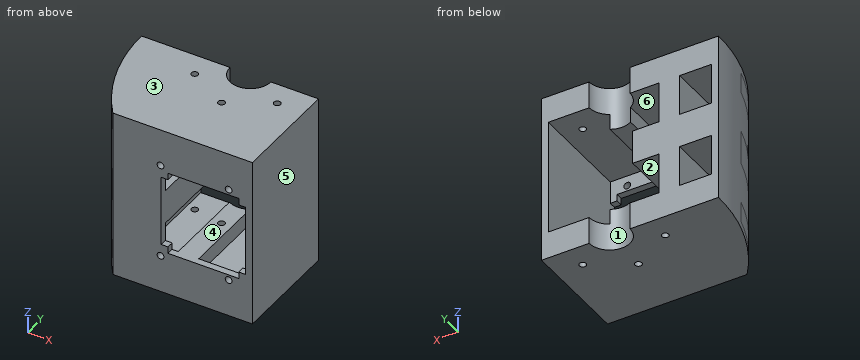
Autodesk Inventor part; units mm, degrees
ref_plane "YZ Plane" through (0, 0, 0) normal (1, 0, 0) x (0, 1, 0)
ref_plane "XZ Plane" through (0, 0, 0) normal (0, 1, 0) x (-1, 0, 0)
ref_plane "XY Plane" through (0, 0, 0) normal (0, 0, 1) x (1, 0, 0)
sketch "Sketch1" plane through (0, 0, 0) normal (0, 0, 1) x (1, 0, 0)
  circle A0 centre (0, 80) radius 130 construction
  line L0 (0, -50) -> (0, 0) construction
  line L1 (0, 0) -> (-102.4695, 0) construction
  arc A1 (-130, 80) -> (-102.4695, 0) centre (0, 80) ccw
  line L2 (-130, 80) -> (0, 80)
  line L3 (0, 80) -> (0, 0)
  line L4 (-102.4695, 0) -> (0, 0)
  dimension "d0" = 260
  dimension "d1" = 50
extrude "Extrusion1" add sketch "Sketch1" along normal blind 125
sketch "Sketch6" plane through (-130, 80, 0) normal (0, 1, 0) x (1, 0, 0)
  line L0 (0, 0) -> (0, -125)
  line L1 (0, 0) -> (130, 0)
  line L2 (130, 0) -> (130, -125)
  line L3 (130, -125) -> (0, -125)
  line L4 (0, -125) -> (0, 0)
  line L5 (5, -120) -> (125, -120)
  line L6 (125, -120) -> (125, -5)
  line L7 (125, -5) -> (5, -5)
  line L8 (5, -5) -> (5, -120)
  point P0 (130, 0)
  dimension "d25" = 5
extrude "Extrusion5" cut sketch "Sketch6" against normal blind 75 contours L8 L7 L6 L5
sketch "Sketch7" plane through (-102.4695, 0, 0) normal (0, -1, 0) x (1, 0, 0)
  circle A0 centre (35, 97.53) radius 2.5
  circle A1 centre (85, 97.53) radius 2.5
  line L0 (0, 125) -> (102.4695, 125)
  line L1 (0, 0) -> (0, 125)
  circle A2 centre (35, 27.53) radius 2.5
  circle A3 centre (85, 27.53) radius 2.5
  line L2 (102.4695, 0) -> (102.4695, 125)
  dimension "d28" = 5
  dimension "d29" = 5
  dimension "d30" = 27.47
  dimension "d31" = 50
  dimension "d33" = 5
  dimension "d34" = 5
  dimension "d35" = 70
  dimension "d82" = 35
extrude "Extrusion6" cut sketch "Sketch7" against normal through all
sketch "Sketch8" plane through (0, 0, 125) normal (0, 0, 1) x (1, 0, 0)
  line L0 (0, 80) -> (-130, 80)
  arc A0 (-130, 80) -> (-102.4695, 0) centre (0, 80) ccw
  arc A1 (-130, 80) -> (-102.4695, 0) centre (9.9581, 83.4269) ccw
  line L1 (-102.4695, 0) -> (-97.4695, 0)
  line L2 (-102.4695, 0) -> (0, 0)
  line L3 (-130, 80) -> (-125, 80)
  arc A2 (-125, 80) -> (-97.4695, 0) centre (14.9581, 83.4269) ccw
  dimension "d40" = 5
  dimension "d41" = 5
  dimension "d42" = 140
extrude "Extrusion7" add sketch "Sketch8" against normal blind 125
sketch "Sketch11" plane through (-130, 5, 0) normal (0, 1, 0) x (1, 0, 0)
  line L0 (125, -5) -> (125, -120)
  line L1 (125, -50) -> (5, -50)
  line L2 (5, -50) -> (5, -65)
  line L3 (5, -65) -> (125, -65)
  line L4 (125, -65) -> (125, -50)
  line L5 (125, -60) -> (5, -60)
  line L6 (5, -60) -> (5, -75)
  line L7 (5, -75) -> (125, -75)
  line L8 (125, -75) -> (125, -60)
  line L9 (32.7619, 0) -> (32.7619, -150)
  line L10 (125, -105) -> (5, -105)
  line L11 (5, -105) -> (5, -120)
  line L12 (5, -120) -> (125, -120)
  line L13 (125, -120) -> (125, -105)
  line L14 (125, -20) -> (5, -20)
  line L15 (5, -20) -> (5, -5)
  line L16 (5, -5) -> (125, -5)
  line L17 (125, -5) -> (125, -20)
  line L18 (5, -5) -> (125, -5)
  line L19 (5, -120) -> (5, -5)
  line L20 (125, -120) -> (5, -120)
  line L21 (125, -5) -> (125, -20)
  point P0 (130, 0)
  point P1 (65, -120)
  point P2 (65, -5)
  point P3 (5, -12.5)
  point P4 (5, -57.5)
  dimension "d54" = 15
  dimension "d55" = 15
  dimension "d56" = 15
  dimension "d57" = 15
  dimension "d58" = 30
  dimension "d59" = 30
  dimension "d66" = 5
extrude "Extrusion10" add sketch "Sketch11" along normal blind 75 contours L0 L14 L9 L16 | L9 L14 L15 L16 | L0 L5 L9 L1 | L0 L3 L9 L5 | L9 L5 L2 L1 | L0 L7 L9 L3 | L9 L3 L2 L5 | L9 L7 L6 L3 | L0 L12 L9 L10 | L9 L12 L11 L10
sketch "Sketch12" plane through (-130, 5, 0) normal (0, 1, 0) x (1, 0, 0)
  line L0 (27.5305, 0) -> (130, 0)
  line L1 (27.5305, -125) -> (130, -125)
  line L2 (72.5, 0) -> (87.5, 0)
  line L3 (87.5, 0) -> (87.5, -125)
  line L4 (87.5, -125) -> (72.5, -125)
  line L5 (72.5, -125) -> (72.5, 0)
  line L6 (28.5256, 0) -> (43.5256, 0)
  line L7 (43.5256, 0) -> (43.5256, -125)
  line L8 (43.5256, -125) -> (28.5256, -125)
  line L9 (28.5256, -125) -> (28.5256, 0)
  line L10 (130, 0) -> (130, -125)
  dimension "d62" = 15
  dimension "d63" = 15
  dimension "d92" = 42.5
extrude "Extrusion11" add sketch "Sketch12" along normal blind 75 contours L0 L7 L1 L9 | L0 L3 L1 L5
sketch "Sketch9" plane through (0, 0, 125) normal (0, 0, 1) x (1, 0, 0)
  circle A0 centre (-50, 80) radius 15
  point P0 (0, 0)
  point P1 (0, 80)
  dimension "d45" = 30
  dimension "d46" = 50
extrude "Extrusion8" cut sketch "Sketch9" against normal through all
sketch "Sketch13" plane through (0, 0, 0) normal (0, 0, -1) x (-1, 0, 0)
  arc A0 (102.4695, 0) -> (130, 80) centre (-9.9581, 83.4269) ccw
  line L0 (130, 80) -> (130, 80)
  arc A1 (102.4695, 0) -> (130, 80) centre (0, 80) ccw
  line L1 (130, 80) -> (130, 80)
  line L2 (65, 80) -> (130, 80)
  line L3 (130, 80) -> (130, 0)
  line L4 (130, 0) -> (102.4695, 0)
  point P0 (0, 0)
  dimension "d67" = 140
extrude "Extrusion12" cut sketch "Sketch13" against normal through all contours A1 L3 L4
sketch "Sketch14" plane through (0, 0, 125) normal (0, 0, 1) x (1, 0, 0)
  line L0 (-102.4695, 0) -> (0, 0) construction
  line L1 (-50, 0) -> (-50, 196.0469) construction
  line L2 (0, 80) -> (-93.0222, 80) construction
  line L3 (-50, 80) -> (28.9192, 80) construction
  circle A0 centre (-50, 115) radius 2.5
  circle A1 centre (-50, 80) radius 35 construction
  circle A2 centre (-80.3109, 97.5) radius 2.5
  circle A3 centre (-80.3109, 62.5) radius 2.5
  circle A4 centre (-50, 45) radius 2.5
  circle A5 centre (-19.6891, 62.5) radius 2.5
  circle A6 centre (-19.6891, 97.5) radius 2.5
  dimension "d74" = 70
  dimension "d70" = 50
  dimension "d72" = 5
  dimension "d77" = 360
extrude "Extrusion13" cut sketch "Sketch14" against normal through all contours A3 | A4 | A5
sketch "Sketch16" plane through (-102.4695, 0, 0) normal (0, -1, 0) x (1, 0, 0)
  line L0 (35.4695, 31.5) -> (35.4695, 93.5) construction
  line L1 (97.4695, 93.5) -> (35.4695, 93.5) construction
  line L2 (35.4695, 93.5) -> (35.4695, 31.5) construction
  line L3 (35.4695, 31.5) -> (97.4695, 31.5) construction
  line L4 (97.4695, 31.5) -> (97.4695, 93.5) construction
  line L5 (0, 125) -> (102.4695, 125)
  line L6 (0, 0) -> (102.4695, 0)
  line L7 (102.4695, 0) -> (102.4695, 125)
  line L8 (97.4695, 93.5) -> (92.4695, 93.5) construction
  line L9 (92.4695, 93.5) -> (92.4695, 88.5) construction
  line L10 (92.4695, 88.5) -> (97.4695, 88.5) construction
  line L11 (97.4695, 88.5) -> (97.4695, 93.5) construction
  line L12 (35.4695, 31.5) -> (40.4695, 31.5) construction
  line L13 (40.4695, 31.5) -> (40.4695, 36.5) construction
  line L14 (40.4695, 36.5) -> (35.4695, 36.5) construction
  line L15 (35.4695, 36.5) -> (35.4695, 31.5) construction
  line L16 (35.4695, 93.5) -> (40.4695, 93.5) construction
  line L17 (40.4695, 93.5) -> (40.4695, 88.5) construction
  line L18 (40.4695, 88.5) -> (35.4695, 88.5) construction
  line L19 (35.4695, 88.5) -> (35.4695, 93.5) construction
  line L20 (97.4695, 31.5) -> (92.4695, 31.5) construction
  line L21 (92.4695, 31.5) -> (92.4695, 36.5) construction
  line L22 (92.4695, 36.5) -> (97.4695, 36.5) construction
  line L23 (97.4695, 36.5) -> (97.4695, 31.5) construction
  line L24 (92.4695, 93.5) -> (40.4695, 93.5)
  line L25 (40.4695, 88.5) -> (40.4695, 93.5)
  line L26 (35.4695, 88.5) -> (40.4695, 88.5)
  line L27 (35.4695, 88.5) -> (35.4695, 36.5)
  line L28 (35.4695, 36.5) -> (40.4695, 36.5)
  line L29 (40.4695, 36.5) -> (40.4695, 31.5)
  line L30 (40.4695, 31.5) -> (92.4695, 31.5)
  line L31 (92.4695, 31.5) -> (92.4695, 36.5)
  line L32 (92.4695, 36.5) -> (97.4695, 36.5)
  line L33 (97.4695, 20) -> (97.4695, 50)
  line L34 (97.4695, 36.5) -> (97.4695, 88.5)
  line L35 (97.4695, 75) -> (97.4695, 105)
  line L36 (92.4695, 88.5) -> (97.4695, 88.5)
  line L37 (92.4695, 88.5) -> (92.4695, 93.5)
  point P0 (97.4695, 62.5)
  point P1 (102.4695, 62.5)
  point P2 (66.4695, 31.5)
  point P3 (51.2348, 0)
  dimension "d100" = 62
  dimension "d101" = 62
  dimension "d102" = 5
  dimension "d103" = 5
  dimension "d104" = 5
  dimension "d105" = 5
  dimension "d106" = 5
  dimension "d107" = 5
  dimension "d108" = 5
  dimension "d109" = 5
  dimension "d110" = 5
extrude "Extrusion15" cut sketch "Sketch16" against normal through all
equation "\"d101\" = d100"
properties part number "SJ005" material "ABS Plastic"
For this review, take the finished solid that the model builds, in its own axes (mm). Face numbers are marked on the shaded views. A direction names the side the tool comes from. Coordinates: 2 decimals unless noted, no trailing zeros. Write each loop counter-clockwise with the first axis right and the second up, starting at its lowest first coordinate (ties: lowest second). Pieces come first, ordered by that corner, then holes. Notation, with made-up numbers: (24.5, 55.5) -> (48.5, 55.5) arc R15 cw to (48.5, 70.5) -> close; hole circle Ø10 at (-8, -25). An arc over 180 degrees is marked (long way). Put each result on its own line as item: value.
Q1. Wall thickness on L1, parallel to Z at x = -75.5, y = 16; L2, parallel to X at y = 16.5, z = 47; L3, parallel to Z at x = -39, y = 65: over which ranges is each line inside the solid? List them lowest first.
From the geometry:
L1: z = 0 to 20, 50 to 75, 105 to 125
L2: x = -113.44 to -108.01, -101.47 to -86.47, -5 to 0
L3: z = 0 to 20, 105 to 125
Q2. Take a section at C-C, the plane z = 45. State the section outline as (x, y) points.
From the geometry:
outline: (-130, 80) arc R130 ccw to (-102.47, 0) -> (-67, 0) -> (-67, 5) -> (-86.47, 5) -> (-86.47, 80) -> (-101.47, 80) -> (-101.47, 5.69) arc R140 cw to (-125, 80) -> close; (-5, 0) -> (0, 0) -> (0, 80) -> (-5, 80) -> close
Q3. Take a section at B-B, the plane x = -50. State the section outline as (y, z) points, then the cut area to 3 significant figures.
From the geometry:
outline: (0, 0) -> (42.5, 0) -> (42.5, 31.5) -> (0, 31.5) -> close; (0, 93.5) -> (42.5, 93.5) -> (42.5, 125) -> (0, 125) -> close; (47.5, 0) -> (65, 0) -> (65, 31.5) -> (47.5, 31.5) -> close; (47.5, 93.5) -> (65, 93.5) -> (65, 125) -> (47.5, 125) -> close
area: 3,780 mm2
Q4. Clearance check with flat-ended pins moving along their axes: pin 1 Ø24 at (y, z) = (56, 53.5) entering from -X; pin 2 Ø10 at (y, z) = (52, 49.5) entering from -X. State where each tip first meets the part, or that it passes through.
From the geometry:
pin 1: stops at x = -129.44
pin 2: stops at x = -127.95
Q5. Tool access review of the marked faces 4, 5 and 6: name each direction out of +Z, -Z, +X, -X, +Y, -Y from which nothing blocks a thin tool from reaching the whole face with its end or side.
From the geometry:
face 4: +Y, -Y
face 5: +Z, -Z, +X, +Y, -Y
face 6: +Y
Q6. Take a section at A-A, the plane z = 97.53. State the section outline as (x, y) points, then the cut area to 3 significant figures.
From the geometry:
outline: (-130, 80) arc R130 ccw to (-102.47, 0) -> (-69.97, 0) -> (-69.97, 5) -> (-86.47, 5) -> (-86.47, 80) -> (-101.47, 80) -> (-101.47, 5.69) arc R140 cw to (-125, 80) -> close; (-64.97, 0) -> (-19.97, 0) -> (-19.97, 5) -> (-42.5, 5) -> (-42.5, 67.01) arc R15 cw to (-57.5, 67.01) -> (-57.5, 5) -> (-64.97, 5) -> close; (-14.97, 0) -> (0, 0) -> (0, 80) -> (-5, 80) -> (-5, 5) -> (-14.97, 5) -> close; hole circle Ø5 at (-50, 45)
area: 3,270 mm2
Q7. The part is to be moulded in two halves that separate along Z. For the marked faces 1, 2 and 3, say which applies: +Z half, -Z half, draft (parallel to the pull), parting line (faces both ways), or undercut.
From the geometry:
face 1: draft
face 2: undercut
face 3: +Z half
Q8. Take a section at D-D, the plane y = 49.5. State the section outline as (x, z) points, then the cut area to 3 significant figures.
From the geometry:
outline: (-126.37, 0) -> (0, 0) -> (0, 125) -> (-126.37, 125) -> close; hole (-120.87, 20) -> (-101.47, 20) -> (-101.47, 50) -> (-120.87, 50) -> close; hole (-120.87, 75) -> (-101.47, 75) -> (-101.47, 105) -> (-120.87, 105) -> close; hole (-86.47, 20) -> (-57.5, 20) -> (-57.5, 31.5) -> (-42.5, 31.5) -> (-42.5, 20) -> (-5, 20) -> (-5, 105) -> (-42.5, 105) -> (-42.5, 93.5) -> (-57.5, 93.5) -> (-57.5, 105) -> (-86.47, 105) -> (-86.47, 75) -> (-67, 75) -> (-67, 50) -> (-86.47, 50) -> close
area: 8,540 mm2
